The listing builds one solid part. Answer for the finished solid, in the listing's coordinates (mm). A direction names the side the tool comes from. Give positions to 0.01 mm unless a question says otherwise; leave off trailing zeros. Order: outer loops, then holes, each group sorted by start corner. A loop starts at its lowest first (then second) coordinate and runs counter-clockwise, first axis right, second up. Notation, with made-up numbers: (62.5, -37) - (98.5, -37) arc R30 cw to (98.5, 2) - close; hole circle Ø10 at (13, -13). An arc over 180 degrees is marked (long way). Answer in a Markdown table with one row per item.
from build123d import *

# Parameters (mm, degrees)
BOSS_EXTRUDE1_DEPTH = 10
SKETCH2_W           = 25
SKETCH2_H           = 55
CUT_EXTRUDE1_DEPTH  = 10


with BuildPart() as part:
    # Sketch1 → Boss-Extrude1 (new body)
    with BuildSketch(Plane(origin=(0, 0, 0), x_dir=(1, 0, 0), z_dir=(0, 1, 0))):
        Polygon((-75, 215), (-75, 0), (75, 0), (75, 215), (85, 215), (85, 315), (75, 315), (75, 560), (25, 560), (25, 121.727049474), (-25, 121.727049474), (-25, 560), (-75, 560), (-75, 315), (-85, 315), (-85, 215), align=None)
    extrude(amount=BOSS_EXTRUDE1_DEPTH)

    # Sketch2 → Cut-Extrude1 (cut)
    with BuildSketch(Plane(origin=(0, 10, 0), x_dir=(1, 0, 0), z_dir=(0, 1, 0))):
        with Locations((62.5, 532.5)):
            Rectangle(SKETCH2_W, SKETCH2_H)
    extrude(amount=-CUT_EXTRUDE1_DEPTH, mode=Mode.SUBTRACT)


solid = part.part
Item 1: Find section C-C on x = -1.5. Write down the section's boundary in (y, z).
Answer block:
| item | result |
|---|---|
| outline | (0, -121.73) - (10, -121.73) - (10, 0) - (0, 0) - close |
Item 2: Consider line 1 (X direction, y = 8, z = -449); line 2 (X direction, y = 1.75, z = -32); line 3 (Z direction, x = 15.5, y = 1.5). Determine where each line is inside the solid, lowest interval first.
Answer block:
| item | result |
|---|---|
| line 1 | -75 to -25, 25 to 75 |
| line 2 | -75 to 75 |
| line 3 | -121.73 to 0 |
Item 3: Find section D-D on z = -291.5. Write down the section's boundary in (x, y), then the cut area to 3 significant figures.
Answer block:
| item | result |
|---|---|
| outline | (-85, 0) - (-25, 0) - (-25, 10) - (-85, 10) - close; (25, 0) - (85, 0) - (85, 10) - (25, 10) - close |
| area | 1,200 mm² |
Item 4: Each of these flat-tipped pins is pushed along its axis until it touches: P1, Ø5, axis at x = -79, y = 5.5, coming from the +Z side; P2, Ø5, axis at y = 5.5, z = -539.5, coming from the +X side; P3, Ø3, axis at x = -79.5, y = 4.5, coming from the -Z side. Where does it stop, or does it pass through?
Answer block:
| item | result |
|---|---|
| P1 | z = -215 |
| P2 | x = 50 |
| P3 | z = -315 |
Item 5: Which of the six approach directions +Z, -Z, +X, -X, +Y, -Y give full straight-line access (tool end or side, diameter ignored) to faces 1 (the face through (75, 5, -106)), 2 (the face through (-80, 5, -315)), 3 (the face through (25, 5, -344)), 4 (the face through (62, 5, -505))?
Answer block:
| item | result |
|---|---|
| face 1 | +Z, +X, +Y, -Y |
| face 2 | -Z, -X, +Y, -Y |
| face 3 | -Z, +Y, -Y |
| face 4 | -Z, +X, +Y, -Y |
Item 6: Find section A-A on z = -411.5. Write down the section's boundary in (x, y), then the cut area to 3 significant figures.
Answer block:
| item | result |
|---|---|
| outline | (-75, 0) - (-25, 0) - (-25, 10) - (-75, 10) - close; (25, 0) - (75, 0) - (75, 10) - (25, 10) - close |
| area | 1,000 mm² |
Item 7: Find section B-B on y = 7.5. Write down the section's boundary in (x, z), then the cut area to 3 significant figures.
Answer block:
| item | result |
|---|---|
| outline | (-85, -315) - (-75, -315) - (-75, -560) - (-25, -560) - (-25, -121.73) - (25, -121.73) - (25, -560) - (50, -560) - (50, -505) - (75, -505) - (75, -315) - (85, -315) - (85, -215) - (75, -215) - (75, 0) - (-75, 0) - (-75, -215) - (-85, -215) - close |
| area | 62,700 mm² |
Item 8: Determine the mould class of faces 5 (the face through (0, 5, -121.727)), 6 (the face through (50, 5, -532)), 7 (the face through (-75, 5, -439)) for opening direction X: pulls with the +X half, pulls with the -X half, needs draft (parallel to the pull), parting line crosses it, or undercut.
Answer block:
| item | result |
|---|---|
| face 5 | undercut |
| face 6 | pulls with the +X half |
| face 7 | pulls with the -X half |
